from build123d import *

# Parameters (mm, degrees)
SKETCH1_W           = 25
SKETCH1_H           = 60
SKETCH1_R           = 3.3
BOSS_EXTRUDE1_DEPTH = 9.5
CHAMFER1_SIZE       = 0.3


with BuildPart() as part:
    # Sketch1 → Boss-Extrude1 (new body)
    with BuildSketch(Plane(origin=(0, 0, 0), x_dir=(1, 0, 0), z_dir=(0, 1, 0))):
        Rectangle(SKETCH1_W, SKETCH1_H)
        with Locations((6.5, 23)):
            Circle(SKETCH1_R, mode=Mode.SUBTRACT)
        with Locations((6.5, -23)):
            Circle(SKETCH1_R, mode=Mode.SUBTRACT)
        with Locations((-6.5, 23)):
            Circle(SKETCH1_R, mode=Mode.SUBTRACT)
        with Locations((-6.5, -23)):
            Circle(SKETCH1_R, mode=Mode.SUBTRACT)
    extrude(amount=BOSS_EXTRUDE1_DEPTH)

    # Chamfer1
    chamfer1_edges = [part.edges().sort_by_distance(p)[0] for p in [
        (-12.5, 4.75, -30),
        (12.5, 4.75, -30),
        (12.5, 4.75, 30),
        (-12.5, 4.75, 30),
    ]]
    chamfer(chamfer1_edges, length=CHAMFER1_SIZE)


solid = part.part
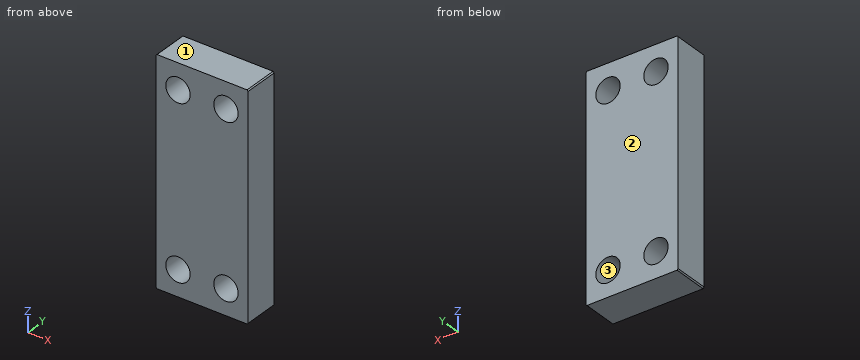
CAD build for the part. Positions are in the model's coordinates, mm. Face numbers are marked on the shaded views. Give positions to 0.01 mm unless a question says otherwise; leave off trailing zeros. Write each loop counter-clockwise with the first axis right and the second up, starting at its lowest first coordinate (ties: lowest second). Pieces come first, ordered by that corner, then holes. Notation, with made-up numbers: (35.5, -29) - (62.5, -29) arc R18 ccw to (62.5, -20) - close; hole circle Ø2 at (38.25, 57). An arc over 180 degrees is marked (long way). Answer as CSV lines item,"result".
Q1. Pull direction Z, two halves, no side cores. Call the marked faces 1, 2 and 3: released by +Z, released by -Z, zero draft, split by the parting line, or undercut.
Result set:
face 1,"released by +Z"
face 2,"zero draft"
face 3,"undercut"
Q2. Drill centre lines: line 1 (X direction, y = 4, z = -23); line 2 (Z direction, x = -6.5, y = 3); line 3 (Z direction, x = 4, y = 2). Where is each one in solid material? Low to high. Write a range as from..to.
Result set:
line 1,"-12.5..-9.8, -3.2..3.2, 9.8..12.5"
line 2,"-30..-26.3, -19.7..19.7, 26.3..30"
line 3,"-30..-25.15, -20.85..20.85, 25.15..30"
Q3. Band-saw the part on A-A (z = -23). Give the cut face in (x, y).
Result set:
outline,"(-12.5, 0) - (-9.8, 0) - (-9.8, 9.5) - (-12.5, 9.5) - close; (-3.2, 0) - (3.2, 0) - (3.2, 9.5) - (-3.2, 9.5) - close; (9.8, 0) - (12.5, 0) - (12.5, 9.5) - (9.8, 9.5) - close"
Q4. Band-saw the part on C-C (x = -6.5). Give the cut face in (y, z), and give its area (3 significant figures).
Result set:
outline,"(0, -30) - (9.5, -30) - (9.5, -26.3) - (0, -26.3) - close; (0, -19.7) - (9.5, -19.7) - (9.5, 19.7) - (0, 19.7) - close; (0, 26.3) - (9.5, 26.3) - (9.5, 30) - (0, 30) - close"
area,"445 mm²"
Q5. Band-saw the part on B-B (y = 4.75). Give the cut face in (x, z).
Result set:
outline,"(-12.5, -29.7) - (-12.2, -30) - (12.2, -30) - (12.5, -29.7) - (12.5, 29.7) - (12.2, 30) - (-12.2, 30) - (-12.5, 29.7) - close; hole circle Ø6.6 at (-6.5, -23); hole circle Ø6.6 at (-6.5, 23); hole circle Ø6.6 at (6.5, -23); hole circle Ø6.6 at (6.5, 23)"
